Job drawing, mm, ordinate dimensions from the low corner. One solid piece. A direction names the side the tool comes from. Give positions to 0.01 mm unless a question says otherwise; leave off trailing zeros. Write each loop counter-clockwise with the first axis right and the second up, starting at its lowest first coordinate (ties: lowest second). Pieces come first, ordered by that corner, then holes. Notation, with made-up numbers: M 58.5,3 L 96.5,3 A20 ccw 96.5,25 Z; hole C -31,39 d3. An arc over 180 degrees is marked long. Use CSV: the item, a comma, the result in double quotes. Start each with the question number.
Item 1: Drill centre lines: line 1 (Y direction, x = 5, z = 19.75); line 2 (Z direction, x = 2, y = 9.25); line 3 (Z direction, x = 1.5, y = 5). Where is each one in solid material? Low to high. Write a range as [from, to].
Item 2: Cut at D-D (y = 5.5). List the corners of the cut face in (x, z), then the cut area to 3 significant figures.
Item 3: Pin check, flat tips, straight feed: pin 1 (4 mm diameter, centred on y = 5.5, z = 7, fed in from -X); pin 2 (4 mm diameter, centred on x = 5, y = 4, fed in from -Z); pin 3 (3.5 mm diameter, centred on x = 5, z = 4, fed in from -Y); pin 4 (5 mm diameter, centred on x = 5, z = 7.5, fed in from +Y). Stop position of each tip, or through.
Item 4: Cut at C-C (z = 5). List the corners of the cut face in (x, y).
Item 5: Which spindle directions (+Z, -Z, +X, -X, +Y, -Y) get a long thin tool onto all of the face, cutting with end or side? Do the marked faces 1, 2, 3, 4 and 5. Say none if no direction does.
Item 6: Cut at A-A (y = 2). List the corners of the cut face in (x, z) (1 decimal).
Item 7: Cut at B-B (x = 8.25). List the corners of the cut face in (y, z) (1 decimal).
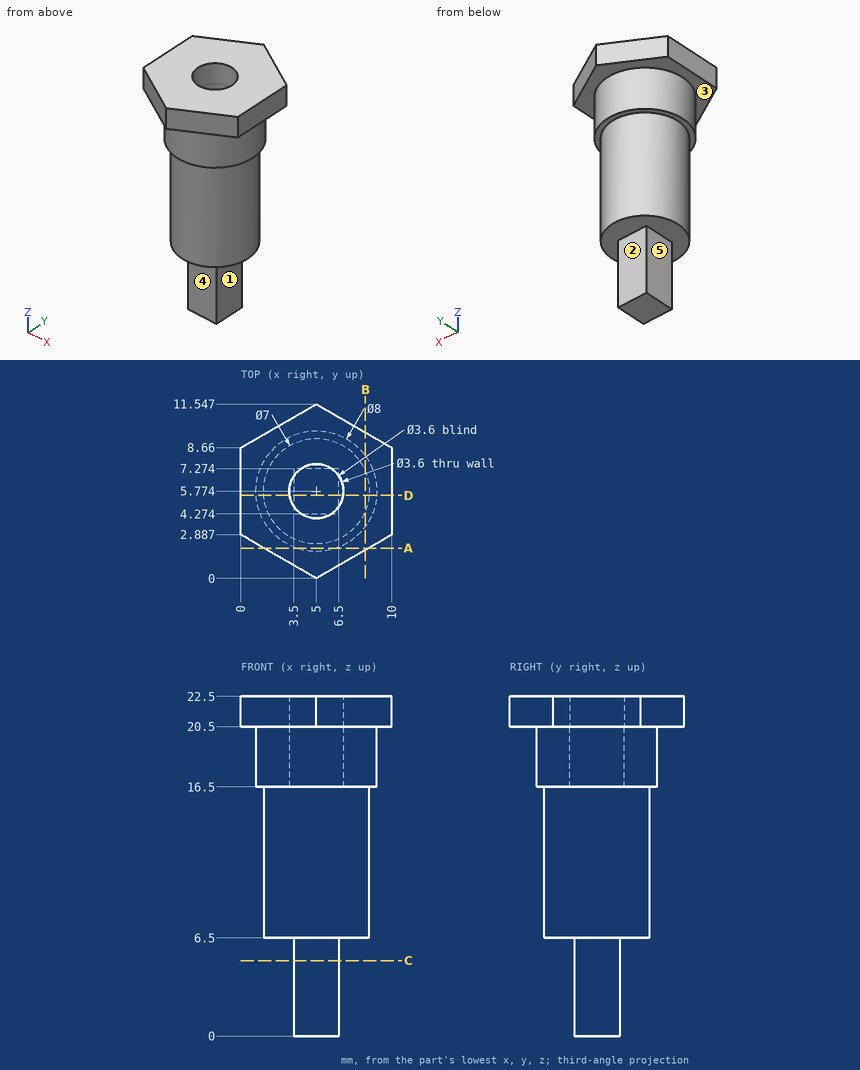
Worked answers:
1,line 1,"y = [1.77, 3.97], [7.57, 9.77]"
1,line 2,"z = [20.5, 22.5]"
1,line 3,"z = [16.5, 22.5]"
2,outline,"M 0,20.5 L 1.01,20.5 L 1.01,16.5 L 1.51,16.5 L 1.51,6.5 L 3.5,6.5 L 3.5,0 L 6.5,0 L 6.5,6.5 L 8.49,6.5 L 8.49,16.5 L 8.99,16.5 L 8.99,20.5 L 10,20.5 L 10,22.5 L 6.78,22.5 L 6.78,16.5 L 3.22,16.5 L 3.22,22.5 L 0,22.5 Z"
2,area,"120 mm^2"
3,pin 1,"stops at x = 1.5"
3,pin 2,"stops at z = 0"
3,pin 3,"stops at y = 4.27"
3,pin 4,"stops at y = 9.27"
4,outline,"M 3.5,4.27 L 6.5,4.27 L 6.5,7.27 L 3.5,7.27 Z"
5,face 1,"-Z, +X, +Y, -Y"
5,face 2,"-Z, +X, -X, +Y"
5,face 3,"-Z"
5,face 4,"-Z, +X, -X, -Y"
5,face 5,"-Z, -X, +Y, -Y"
6,outline,"M 1.5,20.5 L 3.7,20.5 L 3.7,16.5 L 6.3,16.5 L 6.3,20.5 L 8.5,20.5 L 8.5,22.5 L 1.5,22.5 Z"
7,outline,"M 1.9,20.5 L 3.4,20.5 L 3.4,16.5 L 4.5,16.5 L 4.5,6.5 L 7.1,6.5 L 7.1,16.5 L 8.1,16.5 L 8.1,20.5 L 9.7,20.5 L 9.7,22.5 L 1.9,22.5 Z"
